from build123d import *

# Parameters (mm, degrees)
CROQUIS1_W            = 63.5
CROQUIS1_H            = 101.6
BRIDA_BASE1_DEPTH     = 3.4163
CROQUIS2_R            = 6.35
CORTAR_EXTRUIR1_DEPTH = 61.0031133
ROMPER_START          = -3.4163
ROMPER_ESQUINA1_DEPTH = 3.4163


# Read off the part's stored shape, not the designer's step: Romper esquina1
# Sheet-metal steps are written as plain solids
with BuildPart() as part:
    # Croquis1 → Brida base1 (new body)
    with BuildSketch(Plane.XY):
        Rectangle(CROQUIS1_W, CROQUIS1_H)
    extrude(amount=-BRIDA_BASE1_DEPTH)

    # Croquis2 → Cortar-Extruir1 (cut, through all)
    with BuildSketch(Plane.XY):
        with Locations((0, 34.925)):
            Circle(CROQUIS2_R)
        with BuildLine():
            Line((6.35, -31.75), (6.35, -50.8))
            ThreePointArc((6.35, -50.8), (0, -57.15), (-6.35, -50.8))
            Line((-6.35, -50.8), (-6.35, -31.75))
            ThreePointArc((-6.35, -31.75), (0, -25.4), (6.35, -31.75))
        make_face()
    extrude(amount=-CORTAR_EXTRUIR1_DEPTH, mode=Mode.SUBTRACT)

    # Romper esquina1 outline → Romper esquina1 (cut)
    with BuildSketch(Plane.XY.offset(ROMPER_START)):
        with BuildLine():
            Line((6.35, -50.8), (12.7, -50.8))
            ThreePointArc((12.7, -50.8), (8.209871939, -48.940128061), (6.35, -44.45))
            Line((6.35, -44.45), (6.35, -50.8))
        make_face()
        with BuildLine():
            ThreePointArc((-6.35, -44.45), (-8.209871939, -48.940128061), (-12.7, -50.8))
            Line((-12.7, -50.8), (-6.35, -50.8))
            Line((-6.35, -50.8), (-6.35, -44.45))
        make_face()
        with BuildLine():
            ThreePointArc((-25.4, -50.8), (-29.890128061, -48.940128061), (-31.75, -44.45))
            Line((-31.75, -44.45), (-31.75, -50.8))
            Line((-31.75, -50.8), (-25.4, -50.8))
        make_face()
        with BuildLine():
            ThreePointArc((-31.75, 44.45), (-29.890128061, 48.940128061), (-25.4, 50.8))
            Line((-25.4, 50.8), (-31.75, 50.8))
            Line((-31.75, 50.8), (-31.75, 44.45))
        make_face()
        with BuildLine():
            ThreePointArc((25.4, 50.8), (29.890128061, 48.940128061), (31.75, 44.45))
            Line((31.75, 44.45), (31.75, 50.8))
            Line((31.75, 50.8), (25.4, 50.8))
        make_face()
        with BuildLine():
            ThreePointArc((31.75, -44.45), (29.890128061, -48.940128061), (25.4, -50.8))
            Line((25.4, -50.8), (31.75, -50.8))
            Line((31.75, -50.8), (31.75, -44.45))
        make_face()
    extrude(amount=ROMPER_ESQUINA1_DEPTH, mode=Mode.SUBTRACT)


solid = part.part
Can you work these out from the model? Positions are in its coordinate system, mm. A direction names the side the tool comes from. Coordinates: 2 decimals unless noted, no trailing zeros. Write each loop counter-clockwise with the first axis right and the second up, starting at its lowest first coordinate (ties: lowest second). Pieces come first, ordered by that corner, then holes. Notation, with made-up numbers: (66.25, 60.25) -> (72.25, 60.25) arc R31 ccw to (72.25, 98.25) -> close; hole circle Ø5 at (-12, 74.5). An arc over 180 degrees is marked (long way). Write each question's results on one line, items separated by ' | '. Start each with the question number.
Q1. Imagine slicing it at B-B (y = -42.5). Write out the boundary of the cut face in (x, z).
Q2. On a 3-axis mill with a long thin cutter (end or side, diameter ignored), from which of +Z, -Z, +X, -X, +Y, -Y can I reach the whole of each face in a straight line? I mean faces 4 (the face through (0, 50.8, -2)), 5 (the face through (6.35, -38, -2)). Say none if no direction works.
Q3. If I drill on probe 1 along Y at (x, z) = (0, -0.65) (3 decimals); probe 2 along X at (y, z) = (-37, -0.5); probe 3 along X at (y, z) = (33.5, -2.25), over which ranges is the centre line in solid material (lowest first)?
Q4. We'd pull the mould along X, two halves only. Please class faces 1 (the face through (-19, -50.8, -2)), 2 (the face through (-8.16, -48.89, -1.73)), 3 (the face through (31.75, -1, -2)): +X half, -X half, draft (parallel to the pull), parting line (faces both ways), or undercut.
Q5. Imagine slicing it at A-A (x = 0). Write out the boundary of the cut face in (y, z) (3 decimals).
Q6. I'm going to push a flat-ended pin straight in: pin 1 (2 mm diameter, centred on x = 11, z = -3, fed in from -Y). Where does the tip first touch, or does it pass through?
Q7. Imagine slicing it at C-C (z = -2.6). Write out the boundary of the cut face in (x, y) (3 decimals), then the cut area to 3 significant figures.
Taken from the geometry:
1) outline: (-31.75, -3.42) -> (-6.35, -3.42) -> (-6.35, 0) -> (-31.75, 0) -> close; (6.35, -3.42) -> (31.75, -3.42) -> (31.75, 0) -> (6.35, 0) -> close
2) face 4: +Z, -Z, +X, -X, +Y | face 5: +Z, -Z, -Y
3) probe 1: y = -25.4 to 28.575, 41.275 to 50.8 | probe 2: x = -31.75 to -6.35, 6.35 to 31.75 | probe 3: x = -31.75 to -6.19, 6.19 to 31.75
4) face 1: draft | face 2: undercut | face 3: +X half
5) outline: (-25.4, -3.416) -> (28.575, -3.416) -> (28.575, 0) -> (-25.4, 0) -> close; (41.275, -3.416) -> (50.8, -3.416) -> (50.8, 0) -> (41.275, 0) -> close
6) pin 1: stops at y = -50.76
7) outline: (-31.75, -44.45) arc R6.35 ccw to (-25.4, -50.8) -> (-12.7, -50.8) arc R6.35 ccw to (-6.35, -44.45) -> (-6.35, -31.75) arc R6.35 cw to (6.35, -31.75) -> (6.35, -44.45) arc R6.35 ccw to (12.7, -50.8) -> (25.4, -50.8) arc R6.35 ccw to (31.75, -44.45) -> (31.75, 44.45) arc R6.35 ccw to (25.4, 50.8) -> (-25.4, 50.8) arc R6.35 ccw to (-31.75, 44.45) -> close; hole circle Ø12.7 at (0, 34.925) | area: 5,970 mm^2
